Geometry: final body of the model. Coordinates: model frame, mm. Give positions to 0.01 mm unless a question says otherwise; leave off trailing zeros. Loops run counter-clockwise (first coordinate to the right, second up) from the corner with the lowest first, then second, coordinate; pieces in that order, holes last. Notation, with made-up numbers: M 70,-13.5 L 103,-13.5 A24 ccw 103,20.5 Z; hole C -25.75,-17.75 d3. An arc over 180 degrees is marked long. Put each result on its own line as item: value.
```python
from build123d import *

# Parameters (mm, degrees)
SKETCH_1_R          = 1.5
EXTRUDE_1_DEPTH     = 3
SKETCH_2_R          = 1.5
EXTRUDE_2_DEPTH     = 3
EXTRUDE_6_DEPTH     = 3
CUT_EXTRUDE_1_DEPTH = 3
SKETCH_5_R          = 1.5
CUT_EXTRUDE_2_DEPTH = 3
SKETCH_6_R          = 1.5
CUT_EXTRUDE_5_DEPTH = 3
CUT_EXTRUDE_7_DEPTH = 3
CUT_EXTRUDE_9_DEPTH = 3


with BuildPart() as part:
    # 草图1 → 凸台-拉伸1 (new body)
    with BuildSketch(Plane(origin=(0, 0, 0), x_dir=(1, 0, 0), z_dir=(0, 1, 0))):
        Polygon((58, -55), (85, -28), (85, -13.5), (57, -13.5), (57, 13.5), (85, 13.5), (85, 24), (54, 55), (-54, 55), (-85, 24), (-85, 13.5), (-57, 13.5), (-57, -13.5), (-85, -13.5), (-85, -28), (-58, -55), align=None)
        with Locations((77.5, 24)):
            Circle(SKETCH_1_R, mode=Mode.SUBTRACT)
        with Locations((-77.5, 24)):
            Circle(SKETCH_1_R, mode=Mode.SUBTRACT)
        with Locations((-77.5, -24)):
            Circle(SKETCH_1_R, mode=Mode.SUBTRACT)
        with Locations((77.5, -24)):
            Circle(SKETCH_1_R, mode=Mode.SUBTRACT)
    extrude(amount=EXTRUDE_1_DEPTH)

    # 草图2 → 凸台-拉伸2 (add)
    with BuildSketch(Plane(origin=(0, 3, 0), x_dir=(1, 0, 0), z_dir=(0, 1, 0))):
        Polygon((57, 13.5), (85, 13.5), (85, 24), (54.078462186, 54.921537814), (-54.078462186, 54.921537814), (-85, 24), (-85, 13.5), (-57, 13.5), align=None)
        with Locations((-77.5, 24)):
            Circle(SKETCH_2_R, mode=Mode.SUBTRACT)
        with Locations((77.5, 24)):
            Circle(SKETCH_2_R, mode=Mode.SUBTRACT)
        Polygon((-85, 28), (-85, 24), (-54.078462186, 54.921537814), (-58.078462186, 54.921537814), align=None)
        Polygon((54.078462186, 54.921537814), (85, 24), (85, 28), (58.078462186, 54.921537814), align=None)
    extrude(amount=-EXTRUDE_2_DEPTH)

    # 草图3 → 凸台-拉伸6 (add)
    with BuildSketch(Plane.XZ):
        Polygon((-20, 93), (-20, 87.75862069), (20, 122.24137931), (20, 155), (-20, 155), align=None)
        Polygon((20, 122.24137931), (-20, 87.75862069), (-20, 55), (0, 55), (20, 55), (20, 93), align=None)
        Polygon((58, 55), (20, 93), (20, 55), align=None)
        Polygon((-20, 87.75862069), (-58, 55), (-20, 55), align=None)
        Polygon((-20, 93), (-58, 55), (-20, 87.75862069), align=None)
    extrude(amount=-EXTRUDE_6_DEPTH)

    # 草图4 → 切除-拉伸1 (cut)
    with BuildSketch(Plane.XZ):
        with BuildLine():
            Line((37.877062405, -32.043326777), (27.967198456, -32.043326777))
            Line((27.967198456, -32.043326777), (26.920470281, -35.937088984))
            Line((26.920470281, -35.937088984), (34.10030845, -35.937088984))
            ThreePointArc((34.10030845, -35.937088984), (34.626114104, -36.053786172), (34.982522159, -36.457596916))
            Line((34.982522159, -36.457596916), (36.01321058, -38.838842579))
            ThreePointArc((36.01321058, -38.838842579), (36.340515961, -41.403679155), (36.509138095, -43.983811332))
            Line((36.509138095, -43.983811332), (42.601961842, -43.983811332))
            ThreePointArc((42.601961842, -43.983811332), (42.5762659, -39.074399956), (40.794165727, -34.499785293))
            Line((40.794165727, -34.499785293), (45.17492554, -34.499785293))
            ThreePointArc((45.17492554, -34.499785293), (43.76174943, -27.96012409), (38.337690391, -24.04300539))
            Line((38.337690391, -24.04300539), (22.375875232, -24.04300539))
            Line((22.375875232, -24.04300539), (17.015351834, -43.983811332))
            Line((17.015351834, -43.983811332), (22.13492554, -43.983811332))
            Line((22.13492554, -43.983811332), (26.362036193, -28.259228683))
            Line((26.362036193, -28.259228683), (35.785074012, -28.259228683))
            ThreePointArc((35.785074012, -28.259228683), (37.399599712, -29.836972636), (37.877062405, -32.043326777))
        make_face()
        with BuildLine():
            Line((-11.550995986, -24.04300539), (-14.981294936, -36.803499209))
            ThreePointArc((-14.981294936, -36.803499209), (-16.292875485, -38.4823499), (-18.271581685, -39.271973198))
            Line((-18.271581685, -39.271973198), (-23.446816722, -39.271973198))
            Line((-23.446816722, -39.271973198), (-19.251667099, -24.04300539))
            Line((-19.251667099, -24.04300539), (-24.257103323, -24.04300539))
            Line((-24.257103323, -24.04300539), (-27.772258224, -36.803499209))
            ThreePointArc((-27.772258224, -36.803499209), (-28.982580606, -38.443648962), (-30.845065624, -39.271973198))
            Line((-30.845065624, -39.271973198), (-35.909362481, -39.271973198))
            Line((-35.909362481, -39.271973198), (-31.714212859, -24.04300539))
            Line((-31.714212859, -24.04300539), (-36.98159556, -24.04300539))
            Line((-36.98159556, -24.04300539), (-42.474723235, -43.983811332))
            Line((-42.474723235, -43.983811332), (-29.080521508, -43.983811332))
            ThreePointArc((-29.080521508, -43.983811332), (-26.38947659, -42.772882703), (-24.096572177, -40.915287416))
            Line((-24.096572177, -40.915287416), (-24.941863671, -43.983811332))
            Line((-24.941863671, -43.983811332), (-16.438803025, -43.983811332))
            ThreePointArc((-16.438803025, -43.983811332), (-13.277126117, -42.521672977), (-10.843140715, -40.02973307))
            Line((-10.843140715, -40.02973307), (-6.545559762, -24.04300539))
            Line((-6.545559762, -24.04300539), (-11.550995986, -24.04300539))
        make_face()
        with BuildLine():
            Line((0.178860657, -43.983811332), (3.91734543, -30.076885861))
            ThreePointArc((3.91734543, -30.076885861), (3.312428033, -28.889604932), (2.138466003, -28.259228683))
            Line((2.138466003, -28.259228683), (-3.128615616, -28.259228683))
            Line((-3.128615616, -28.259228683), (-1.99520287, -24.04300539))
            Line((-1.99520287, -24.04300539), (13.155847737, -24.04300539))
            ThreePointArc((13.155847737, -24.04300539), (15.376465747, -25.688977693), (16.393411668, -28.259228683))
            Line((16.393411668, -28.259228683), (9.435065309, -28.259228683))
            Line((9.435065309, -28.259228683), (9.435065309, -29.158996281))
            Line((9.435065309, -29.158996281), (5.449831804, -43.983811332))
            Line((5.449831804, -43.983811332), (0.178860657, -43.983811332))
        make_face()
    extrude(amount=-CUT_EXTRUDE_1_DEPTH, mode=Mode.SUBTRACT)

    # 草图5 → 切除-拉伸2 (cut)
    with BuildSketch(Plane.XZ):
        with Locations((45, 55)):
            Circle(SKETCH_5_R)
        with Locations((-45, 55)):
            Circle(SKETCH_5_R)
        with Locations((20, 55)):
            Circle(SKETCH_5_R)
        with Locations((-20, 55)):
            Circle(SKETCH_5_R)
        with Locations((45, 45)):
            Circle(SKETCH_5_R)
        with Locations((-45, 45)):
            Circle(SKETCH_5_R)
        with Locations((-45, 0)):
            Circle(SKETCH_5_R)
        with Locations((45, 0)):
            Circle(SKETCH_5_R)
        with Locations((45, -10)):
            Circle(SKETCH_5_R)
        with Locations((-45, -10)):
            Circle(SKETCH_5_R)
        with Locations((20, 0)):
            Circle(SKETCH_5_R)
        with Locations((-20, 0)):
            Circle(SKETCH_5_R)
        with Locations((20, -10)):
            Circle(SKETCH_5_R)
        with Locations((-20, -10)):
            Circle(SKETCH_5_R)
    extrude(amount=-CUT_EXTRUDE_2_DEPTH, mode=Mode.SUBTRACT)

    # 草图6 → 切除-拉伸5 (cut)
    with BuildSketch(Plane.XZ):
        with BuildLine():
            Line((0, 150.5), (0, 152))
            Line((0, 152), (-9.5, 152))
            ThreePointArc((-9.5, 152), (-8.439339828, 151.560660172), (-8, 150.5))
            Line((-8, 150.5), (0, 150.5))
        make_face()
        with BuildLine():
            Line((0, 149), (0, 150.5))
            Line((0, 150.5), (-8, 150.5))
            ThreePointArc((-8, 150.5), (-8.439339828, 149.439339828), (-9.5, 149))
            Line((-9.5, 149), (0, 149))
        make_face()
        with BuildLine():
            ThreePointArc((-8, 150.5), (-8.439339828, 151.560660172), (-9.5, 152))
            ThreePointArc((-9.5, 152), (-10.560660172, 151.560660172), (-11, 150.5))
            Line((-11, 150.5), (-8, 150.5))
        make_face()
        with BuildLine():
            ThreePointArc((-9.5, 149), (-8.439339828, 149.439339828), (-8, 150.5))
            Line((-8, 150.5), (-11, 150.5))
            ThreePointArc((-11, 150.5), (-10.560660172, 149.439339828), (-9.5, 149))
        make_face()
        with BuildLine():
            Line((9.5, 152), (0, 152))
            Line((0, 152), (0, 150.5))
            Line((0, 150.5), (8, 150.5))
            ThreePointArc((8, 150.5), (8.439339828, 151.560660172), (9.5, 152))
        make_face()
        with BuildLine():
            Line((8, 150.5), (0, 150.5))
            Line((0, 150.5), (0, 149))
            Line((0, 149), (9.5, 149))
            ThreePointArc((9.5, 149), (8.439339828, 149.439339828), (8, 150.5))
        make_face()
        with BuildLine():
            ThreePointArc((11, 150.5), (10.560660172, 151.560660172), (9.5, 152))
            ThreePointArc((9.5, 152), (8.439339828, 151.560660172), (8, 150.5))
            Line((8, 150.5), (9.5, 150.5))
            Line((9.5, 150.5), (11, 150.5))
        make_face()
        with BuildLine():
            Line((9.5, 150.5), (8, 150.5))
            ThreePointArc((8, 150.5), (8.439339828, 149.439339828), (9.5, 149))
            ThreePointArc((9.5, 149), (10.560660172, 149.439339828), (11, 150.5))
            Line((11, 150.5), (9.5, 150.5))
        make_face()
        with Locations((0, 140.5)):
            Circle(SKETCH_6_R)
        with Locations((-15.5, 150.5)):
            Circle(SKETCH_6_R)
        with Locations((15.5, 150.5)):
            Circle(SKETCH_6_R)
    extrude(amount=-CUT_EXTRUDE_5_DEPTH, mode=Mode.SUBTRACT)

    # 草图7 → 切除-拉伸7 (cut)
    with BuildSketch(Plane.XZ):
        with BuildLine():
            ThreePointArc((-8, 131), (-9.414213562, 130.414213562), (-10, 129))
            Line((-10, 129), (-10, 98.857864376))
            ThreePointArc((-10, 98.857864376), (-9.414213562, 97.443650814), (-8, 96.857864376))
            Line((-8, 96.857864376), (8, 96.857864376))
            ThreePointArc((8, 96.857864376), (9.414213562, 97.443650814), (10, 98.857864376))
            Line((10, 98.857864376), (10, 129))
            ThreePointArc((10, 129), (9.414213562, 130.414213562), (8, 131))
            Line((8, 131), (-8, 131))
        make_face()
        with BuildLine():
            Line((10, 88.857864376), (-10, 88.857864376))
            Line((-10, 88.857864376), (-30.943650814, 67.914213562))
            ThreePointArc((-30.943650814, 67.914213562), (-31.377196317, 65.734633135), (-29.529437252, 64.5))
            Line((-29.529437252, 64.5), (29.529437252, 64.5))
            ThreePointArc((29.529437252, 64.5), (31.377196317, 65.734633135), (30.943650814, 67.914213562))
            Line((30.943650814, 67.914213562), (10, 88.857864376))
        make_face()
    extrude(amount=-CUT_EXTRUDE_7_DEPTH, mode=Mode.SUBTRACT)

    # 草图8 → 切除-拉伸9 (cut)
    with BuildSketch(Plane.XZ):
        with BuildLine():
            Line((31.529437252, 38.5), (31.529437252, 16.5))
            ThreePointArc((31.529437252, 16.5), (30.064971157, 12.964466094), (26.529437252, 11.5))
            Line((26.529437252, 11.5), (-26.529437252, 11.5))
            ThreePointArc((-26.529437252, 11.5), (-30.064971157, 12.964466094), (-31.529437252, 16.5))
            Line((-31.529437252, 16.5), (-31.529437252, 38.5))
            ThreePointArc((-31.529437252, 38.5), (-30.064971157, 42.035533906), (-26.529437252, 43.5))
            Line((-26.529437252, 43.5), (26.529437252, 43.5))
            ThreePointArc((26.529437252, 43.5), (30.064971157, 42.035533906), (31.529437252, 38.5))
        make_face()
    extrude(amount=-CUT_EXTRUDE_9_DEPTH, mode=Mode.SUBTRACT)


solid = part.part
```
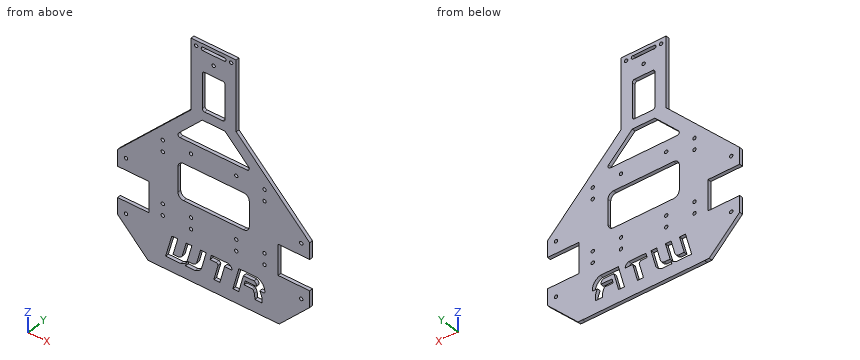
Item 1: Section C-C on y = 1.2. Count the separate pieces of the cut face and the enclosed holes in it, then the cut area to 3 significant figures.
Output values:
separate pieces: 1
enclosed holes: 28
area: 16,400 mm²
Item 2: Section A-A on x = -67.5. Output: boundary loops of the cut face in (y, z).
Output values:
outline: M 0,-45.5 L 3,-45.5 L 3,-13.5 L 0,-13.5 Z; M 0,13.5 L 3,13.5 L 3,45.5 L 0,45.5 Z
Item 3: Pin query (flat end, axial travel): pin 1 Ø4 at (x, z) = (-45, -10) entering from +Y; pin 2 Ø1.5 at (y, z) = (2.5, 113.5) entering from -X; pin 3 Ø1.8 at (x, z) = (45, 45) entering from -Y; pin 4 Ø1.5 at (y, z) = (2, 112) entering from +X. Return the tip coordinate at first contact, or that it passes through.
Output values:
pin 1: y = 3
pin 2: x = -20
pin 3: through
pin 4: x = 20
Item 4: Line query: probe 1 along Z at (x, y) = (-6, 1.15); probe 2 along X at (y, z) = (1.05, -24); probe 3 along Z at (x, y) = (-78, 1.9). Output: solid intervals per line, ascending. Write a range as [from, to].
Output values:
probe 1: [-55, 11.5], [43.5, 64.5], [88.86, 96.86], [131, 149], [152, 155]
probe 2: [-85, -79], [-76, 76], [79, 85]
probe 3: [-35, -25.41], [-22.59, -13.5], [13.5, 22.59], [25.41, 35]
Item 5: Section B-B on z = 118. Output: boundary loops of the cut face in (x, y), then the cut area to 3 significant figures.
Output values:
outline: M -20,0 L -10,0 L -10,3 L -20,3 Z; M 10,0 L 20,0 L 20,3 L 10,3 Z
area: 60.0 mm²
